The listing builds one solid part. Answer for the finished solid, in the listing's coordinates (mm). A direction names the side the tool comes from. Coordinates: 2 decimals unless noted, no trailing zeros. Order: outer loops, then holes, each group sorted by start corner. A loop starts at its lowest first (then second) coordinate and runs counter-clockwise, first axis right, second up. Notation, with made-up numbers: (-28, 57) - (15, 57) arc R30 cw to (15, 95) - close; hole circle Ø5 at (33.5, 81.25). An arc over 180 degrees is marked (long way). Use one line per item in the form item = value. Start each with the question number.
Item 1: Section D-D, the plane x = -0.5 is taken. Write down the section's boundary in (y, z), and give its area (3 significant figures).
Item 2: Consider line 1 along Y through (x, z) = (-25.8, -1.15); line 2 along Y through (x, z) = (17.5, -1.95); line 3 along Y through (x, z) = (12.5, -3). Determine where each line is inside the solid, lowest interval first. Write a range as [from, to].
Item 3: Section B-B, the plane y = -10 is taken. Write down the section's boundary in (x, z), and give its area (3 significant figures).
Item 4: Each of these flat-tipped pins is pushed along its axis until it touches: pin 1 Ø2 at (x, y) = (10, -12) entering from -Z; pin 2 Ø1.3 at (x, y) = (11, 19) entering from -Z. Where does it stop, or does it pass through?
Item 5: Section A-A, the plane x = 10.2 is taken. Write down the section's boundary in (y, z), and give its area (3 significant figures).
Item 6: The mould has two halves that part along X. Classify faces 3 (the cylindrical face through (-23.544, 19.634, -2.578)), 4 (the flat face through (-29.7, 0, -3)), 5 (the cylindrical face through (29.13, -21.1, -2.96)): released by +X, released by -X, zero draft, split by the parting line, or undercut.
Item 7: Section C-C, the plane z = -3.45 is taken. Count the separate pieces of the cut face and the enclosed holes in it, and give its area (3 significant figures).
Item 8: A tool of negligible diameter and unlimited length cuts with its end or side. For faces 1 (the flat face through (0, 0, 0)), 2 (the cylindrical face through (-23.521, -19.663, -2.578)), from which of +Z, -Z, +X, -X, +Y, -Y can it reach the whole face along a straight path? Write none if from no direction.
from build123d import *

# Parameters (mm, degrees)
SKETCH_1_W          = 59.4
SKETCH_1_H          = 43.4
EXTRUDE_1_DEPTH     = 6
SKETCH_2_W          = 56.4
SKETCH_2_H          = 40.4
CUT_EXTRUDE_1_DEPTH = 5
EXTRUDE_2_DEPTH     = 3.2
EXTRUDE_3_DEPTH     = 3.2
EXTRUDE_4_DEPTH     = 3.2
EXTRUDE_5_DEPTH     = 3.2
FILLET_1_R          = 1
FILLET_2_R          = 2
SKETCH_7_R          = 1.45
CUT_EXTRUDE_2_DEPTH = 20


with BuildPart() as part:
    # 草图1 → 凸台-拉伸1 (new body)
    with BuildSketch(Plane(origin=(0, 0, -6), x_dir=(-1, 0, 0), z_dir=(0, 0, -1))):
        Rectangle(SKETCH_1_W, SKETCH_1_H)
    extrude(amount=-EXTRUDE_1_DEPTH)

    # 草图2 → 切除-拉伸1 (cut)
    with BuildSketch(Plane(origin=(0, 0, -6), x_dir=(-1, 0, 0), z_dir=(0, 0, -1))):
        Rectangle(SKETCH_2_W, SKETCH_2_H)
    extrude(amount=-CUT_EXTRUDE_1_DEPTH, mode=Mode.SUBTRACT)

    # 草图3 → 凸台-拉伸2 (add)
    with BuildSketch(Plane(origin=(0, 0, -1), x_dir=(-1, 0, 0), z_dir=(0, 0, -1))):
        with BuildLine():
            Line((-13.62928564, 20.2), (-6.77071436, 20.2))
            ThreePointArc((-6.77071436, 20.2), (-7.932609364, 19.648683298), (-8.240408206, 18.4))
            ThreePointArc((-8.240408206, 18.4), (-10.2, 16), (-12.159591794, 18.4))
            ThreePointArc((-12.159591794, 18.4), (-12.467390636, 19.648683298), (-13.62928564, 20.2))
        make_face()
    extrude(amount=EXTRUDE_2_DEPTH)

    # 草图4 → 凸台-拉伸3 (add)
    with BuildSketch(Plane(origin=(0, 0, -1), x_dir=(-1, 0, 0), z_dir=(0, 0, -1))):
        with BuildLine():
            Line((22.37071436, 20.2), (28.2, 20.2))
            Line((28.2, 20.2), (28.2, 14.617693095))
            ThreePointArc((28.2, 14.617693095), (27.6141741, 15.806930546), (26.314285714, 16.067253197))
            ThreePointArc((26.314285714, 16.067253197), (24.427901488, 16.544889808), (23.840408206, 18.4))
            ThreePointArc((23.840408206, 18.4), (23.532609364, 19.648683298), (22.37071436, 20.2))
        make_face()
    extrude(amount=EXTRUDE_3_DEPTH)

    # 草图5 → 凸台-拉伸4 (add)
    with BuildSketch(Plane(origin=(0, 0, -1), x_dir=(-1, 0, 0), z_dir=(0, 0, -1))):
        with BuildLine():
            Line((28.2, -14.617693095), (28.2, -20.2))
            Line((28.2, -20.2), (22.37071436, -20.2))
            ThreePointArc((22.37071436, -20.2), (23.532609364, -19.648683298), (23.840408206, -18.4))
            ThreePointArc((23.840408206, -18.4), (24.427901488, -16.544889808), (26.314285714, -16.067253197))
            ThreePointArc((26.314285714, -16.067253197), (27.6141741, -15.806930546), (28.2, -14.617693095))
        make_face()
    extrude(amount=EXTRUDE_4_DEPTH)

    # 草图6 → 凸台-拉伸5 (add)
    with BuildSketch(Plane(origin=(0, 0, -1), x_dir=(-1, 0, 0), z_dir=(0, 0, -1))):
        with BuildLine():
            Line((-6.77071436, -20.2), (-13.62928564, -20.2))
            ThreePointArc((-13.62928564, -20.2), (-12.467390636, -19.648683298), (-12.159591794, -18.4))
            ThreePointArc((-12.159591794, -18.4), (-10.2, -16), (-8.240408206, -18.4))
            ThreePointArc((-8.240408206, -18.4), (-7.932609364, -19.648683298), (-6.77071436, -20.2))
        make_face()
    extrude(amount=EXTRUDE_5_DEPTH)

    # 圆角1
    fillet_1_edges = [part.edges().sort_by_distance(p)[0] for p in [
        (28.2, -20.2, -3.5),
        (28.2, 20.2, -3.5),
        (-28.2, 20.2, -5.1),
        (-28.2, -20.2, -5.1),
    ]]
    fillet(fillet_1_edges, radius=FILLET_1_R)

    # 圆角2
    fillet_2_edges = [part.edges().sort_by_distance(p)[0] for p in [
        (-29.7, 21.7, -3),
        (-29.7, -21.7, -3),
        (29.7, -21.7, -3),
        (29.7, 21.7, -3),
    ]]
    fillet(fillet_2_edges, radius=FILLET_2_R)

    # 草图7 → 切除-拉伸2 (cut)
    with BuildSketch(Plane(origin=(0, 0, -4.2), x_dir=(-1, 0, 0), z_dir=(0, 0, -1))):
        with Locations((-10.2, 18)):
            Circle(SKETCH_7_R)
        with Locations((-10.2, -18)):
            Circle(SKETCH_7_R)
        with Locations((25.8, 18)):
            Circle(SKETCH_7_R)
        with Locations((25.8, -18)):
            Circle(SKETCH_7_R)
    extrude(amount=-CUT_EXTRUDE_2_DEPTH, mode=Mode.SUBTRACT)


solid = part.part
Response:
q1.outline = (-21.7, -6) - (-20.2, -6) - (-20.2, -1) - (20.2, -1) - (20.2, -6) - (21.7, -6) - (21.7, 0) - (-21.7, 0) - close
q1.area = 58.4 mm2
q2.line_1 = [-21.7, -19.45], [-16.55, -16], [16, 16.55], [19.45, 21.7]
q2.line_2 = [-21.7, -20.2], [20.2, 21.7]
q2.line_3 = [-21.7, -19.69], [19.69, 21.7]
q3.outline = (-29.7, -6) - (-28.2, -6) - (-28.2, -1) - (28.2, -1) - (28.2, -6) - (29.7, -6) - (29.7, 0) - (-29.7, 0) - close
q3.area = 74.4 mm2
q4.pin_1 = -1
q4.pin_2 = -4.2
q5.outline = (-21.7, -6) - (-20.2, -6) - (-20.2, -4.2) - (-19.45, -4.2) - (-19.45, 0) - (-21.7, 0) - close; (-16.55, -4.2) - (-16, -4.2) - (-16, -1) - (16, -1) - (16, -4.2) - (16.55, -4.2) - (16.55, 0) - (-16.55, 0) - close; (19.45, -4.2) - (20.2, -4.2) - (20.2, -6) - (21.7, -6) - (21.7, 0) - (19.45, 0) - close
q5.area = 60.9 mm2
q6.face_3 = undercut
q6.face_4 = released by -X
q6.face_5 = released by +X
q7.separate_pieces = 1
q7.enclosed_holes = 5
q7.area = 338 mm2
q8.face_1 = +Z, +X, -X, +Y, -Y
q8.face_2 = -Z
